Can you work these out from the model? Positions are in its coordinate system, mm. A direction names the side the tool comes from. Coordinates: 2 decimals unless noted, no trailing zeros. Loops run counter-clockwise (first coordinate to the right, second up) from the corner with the lowest first, then second, coordinate; pieces in that order, holes last. Notation, with made-up numbers: (59.25, 54.25) -> (108.25, 54.25) arc R18 ccw to (108.25, 79.25) -> close; hole circle Ø9 at (-18, -37). An arc over 180 degrees is marked (long way). Put each result on its own line as item: value. Start each with the question number.
Item 1: If we section it at D-D on z = 0: Please give me the cut outline in (x, y) (3 decimals), plus the area to 3 significant figures.
Item 2: For faces 1 (the cylindrical face through (-0.69, -68.2, -3.1)), 2 (the flat face through (28.2, -28, 0)), which set-ups out of +Z, -Z, +X, -X, +Y, -Y let a thin tool reach every point of the face, with its end or its side?
Item 3: If we section it at C-C on x = 23.57: Please give me the cut outline in (y, z), plus the area to 3 significant figures.
Item 4: Will these pins go through, and if not, where does the flat tip stop? P1, Ø2, axis at x = -20.5, z = 2.5, coming from the -Y side; P2, Ø3, axis at x = -23.57, z = 23.57, coming from the -Y side; P3, Ø6, axis at x = -6.5, z = -3.5, coming from the -Y side.
Item 5: Please list where these lines run through material, in increasing order: L1, parallel to Z at x = 23.57, y = -23.5; L2, parallel to X at y = -32, z = -23. Write a range as from..to.
Item 6: If we section it at A-A on y = -28.5: Please give me the cut outline in (x, z).
Item 7: We'd pull the mould along Z, two halves only. Please class faces 3 (the flat face through (-26.91, -27.61, -26.95)), 4 (the flat face through (4, -57.6, 0)), 5 (the cylindrical face through (-21.73, -27.61, 25.26)): pulls with the +Z half, pulls with the -Z half, needs draft (parallel to the pull), parting line crosses it, or undercut.
Item 8: If we section it at B-B on z = 23.57: Please give me the cut outline in (x, y).
```python
from build123d import *

# Parameters (mm, degrees)
F0_W     = 56.4
F0_H     = 56.4
F1_DEPTH = 56
F2_R     = 19.05
F3_DEPTH = 1.6
F4_R     = 3.175
F5_DEPTH = 21.5
F6_R     = 2.5
F7_DEPTH = 79.101
F8_SIZE  = 2.54


with BuildPart() as f1:
    # F0 (on Front) → F1 (new body)
    with BuildSketch(Plane.XZ):
        Rectangle(F0_W, F0_H)
    extrude(amount=F1_DEPTH)

    # F2 (on face) → F3 (join)
    with BuildSketch(Plane.XZ.offset(56)):
        Circle(F2_R)
    extrude(amount=F3_DEPTH)

    # F4 (on face) → F5 (join)
    with BuildSketch(Plane.XZ.offset(57.6)):
        Circle(F4_R)
    extrude(amount=F5_DEPTH)

    # F6 (on face) → F7 (cut, through all)
    with BuildSketch(Plane(origin=(0, 0, 0), x_dir=(-1, 0, 0), z_dir=(0, 1, 0))):
        with Locations((23.57, 23.57)):
            Circle(F6_R)
        with Locations((23.57, -23.57)):
            Circle(F6_R)
        with Locations((-23.57, -23.57)):
            Circle(F6_R)
        with Locations((-23.57, 23.57)):
            Circle(F6_R)
    extrude(amount=-F7_DEPTH, mode=Mode.SUBTRACT)

    # F8
    f8_edges = [f1.edges().sort_by_distance(p)[0] for p in [
        (28.2, -28, 28.2),
        (-28.2, -28, 28.2),
        (-28.2, -28, -28.2),
        (28.2, -28, -28.2),
    ]]
    chamfer(f8_edges, length=F8_SIZE)


solid = f1.part
```
Solutions:
1. outline: (-28.2, -56) -> (-19.05, -56) -> (-19.05, -57.6) -> (-3.175, -57.6) -> (-3.175, -79.1) -> (3.175, -79.1) -> (3.175, -57.6) -> (19.05, -57.6) -> (19.05, -56) -> (28.2, -56) -> (28.2, 0) -> (-28.2, 0) -> close
1. area: 3,360 mm^2
2. face 1: -Y
2. face 2: +Z, -Z, +X, +Y, -Y
3. outline: (-56, -28.2) -> (0, -28.2) -> (0, -26.07) -> (-56, -26.07) -> close; (-56, -21.07) -> (0, -21.07) -> (0, 21.07) -> (-56, 21.07) -> close; (-56, 26.07) -> (0, 26.07) -> (0, 28.2) -> (-56, 28.2) -> close
3. area: 2,600 mm^2
4. P1: y = -56
4. P2: through
4. P3: y = -57.6
5. L1: -28.2..-26.07, -21.07..21.07, 26.07..28.2
5. L2: -28.2..-26, -21.14..21.14, 26..28.2
6. outline: (-28.2, -25.66) -> (-25.66, -28.2) -> (25.66, -28.2) -> (28.2, -25.66) -> (28.2, 25.66) -> (25.66, 28.2) -> (-25.66, 28.2) -> (-28.2, 25.66) -> close; hole circle Ø5 at (-23.57, -23.57); hole circle Ø5 at (-23.57, 23.57); hole circle Ø5 at (23.57, -23.57); hole circle Ø5 at (23.57, 23.57)
7. face 3: pulls with the -Z half
7. face 4: needs draft
7. face 5: undercut
8. outline: (-28.2, -56) -> (-26.07, -56) -> (-26.07, 0) -> (-28.2, 0) -> close; (-21.07, -56) -> (21.07, -56) -> (21.07, 0) -> (-21.07, 0) -> close; (26.07, -56) -> (28.2, -56) -> (28.2, 0) -> (26.07, 0) -> close
